Geometry: final body of the model. Coordinates: model frame, mm. A direction names the side the tool comes from. Give positions to 0.01 mm unless a question says otherwise; leave off trailing zeros. Loops run counter-clockwise (first coordinate to the right, second up) from the corner with the lowest first, then second, coordinate; pieces in that order, holes last. Notation, with made-up numbers: (56, -37.75) - (74, -37.75) arc R26 cw to (74, -16.75) - close; hole circle Ø11 at (18, -26.75). An arc over 180 degrees is marked (long way). Answer in a Markdown table with one row per item.
from build123d import *

# Parameters (mm, degrees)
BOSS_EXTRUDE2_DEPTH    = 4
SKETCH4_W              = 35
SKETCH4_H              = 4
BOSS_EXTRUDE3_DEPTH    = 10
BOSS_EXTRUDE4_DEPTH    = 35
SKETCH9_R              = 2.5
CUT_EXTRUDE1_DEPTH     = 6
SKETCH10_R             = 1.25
CUT_EXTRUDE2_DEPTH     = 6
SKETCH11_R             = 2.5
CUT_EXTRUDE3_DEPTH     = 4
CONVERT_SOLID2_START   = -17.5
CONVERT_SOLID2_DEPTH   = 35
CONVERT_SOLID2_2_DEPTH = 35
CONVERT_SOLID2_3_DEPTH = 15
CONVERT_SOLID2_START_2 = 2.5
CONVERT_SOLID2_4_DEPTH = 15


# Read off the part's stored shape, not the designer's step: Convert-Solid2
with BuildPart() as part:
    # Sketch3 → Boss-Extrude2 (new body)
    with BuildSketch(Plane(origin=(0, 0, 0), x_dir=(1, 0, 0), z_dir=(0, 1, 0))):
        with BuildLine():
            Line((-17.5, 0), (-17.5, 27.5))
            Line((-17.5, 27.5), (17.5, 27.5))
            Line((17.5, 27.5), (17.5, 0))
            ThreePointArc((17.5, 0), (0, -17.5), (-17.5, 0))
        make_face()
    extrude(amount=BOSS_EXTRUDE2_DEPTH)

    # Sketch4 → Boss-Extrude3 (add)
    with BuildSketch(Plane(origin=(0, 4, 0), x_dir=(1, 0, 0), z_dir=(0, 1, 0))):
        with Locations((0, 25.5)):
            Rectangle(SKETCH4_W, SKETCH4_H)
    extrude(amount=BOSS_EXTRUDE3_DEPTH)

    # Sketch6 → Boss-Extrude4 (add)
    with BuildSketch(Plane.ZY.offset(17.5)):
        Polygon((-27.5, 14), (-27.5, 18), (-2.5, 18), (-2.5, 128), (1.5, 128), (1.5, 14), align=None)
    extrude(amount=-BOSS_EXTRUDE4_DEPTH)

    # Sketch9 → Cut-Extrude1 (cut)
    with BuildSketch(Plane.XY.offset(1.5)):
        with Locations((-8.9, 117.2)):
            Circle(SKETCH9_R)
        with Locations(Location((8.9, 117.2, 0), (0, 0, 180))):
            Circle(SKETCH9_R)
        with Locations(Location((-8.9, 42.7, 0), (0, 0, 180))):
            Circle(SKETCH9_R)
        with Locations((8.9, 42.7)):
            Circle(SKETCH9_R)
        Polygon((-15.1, 113), (-2.5, 113), (-2.5, 125.287895972), (0, 125.287895972), (2.5, 125.287895972), (2.5, 113), (15.1, 113), (15.1, 46.9), (2.5, 46.9), (2.5, 10), (-2.5, 10), (-2.5, 46.9), (-15.1, 46.9), align=None)
    extrude(amount=-CUT_EXTRUDE1_DEPTH, mode=Mode.SUBTRACT)

    # Sketch10 → Cut-Extrude2 (cut)
    with BuildSketch(Plane.XZ):
        with Locations(Location((-8.75, 0, 0), (0, 0, 270))):
            Circle(SKETCH10_R)
        with Locations(Location((8.75, 0, 0), (0, 0, 90))):
            Circle(SKETCH10_R)
        with Locations(Location((0, 8.75, 0), (0, 0, 270))):
            Circle(SKETCH10_R)
        with Locations(Location((0, -8.75, 0), (0, 0, 270))):
            Circle(SKETCH10_R)
    extrude(amount=-CUT_EXTRUDE2_DEPTH, mode=Mode.SUBTRACT)

    # Sketch11 → Cut-Extrude3 (cut)
    with BuildSketch(Plane.XZ):
        with Locations(Location((0, 0, 0), (0, 0, 270))):
            Circle(SKETCH11_R)
    extrude(amount=-CUT_EXTRUDE3_DEPTH, mode=Mode.SUBTRACT)

    # Convert-Solid2 outline → Convert-Solid2 (cut)
    with BuildSketch(Plane.YZ.offset(CONVERT_SOLID2_START)):
        with BuildLine():
            Line((0, -27.5), (4.1, -27.5))
            ThreePointArc((4.1, -27.5), (1.200862197, -26.299137803), (0, -23.4))
            Line((0, -23.4), (0, -27.5))
        make_face()
        with BuildLine():
            Line((18, -27.5), (18, -23.4))
            ThreePointArc((18, -23.4), (16.799137803, -26.299137803), (13.9, -27.5))
            Line((13.9, -27.5), (18, -27.5))
        make_face()
        with BuildLine():
            ThreePointArc((14, -2.6), (15.200862197, 0.299137803), (18.1, 1.5))
            Line((18.1, 1.5), (14, 1.5))
            Line((14, 1.5), (14, -2.6))
        make_face()
    extrude(amount=CONVERT_SOLID2_DEPTH, mode=Mode.SUBTRACT)

    # Convert-Solid2 2 outline → Convert-Solid2 2 (add)
    with BuildSketch(Plane.YZ.offset(CONVERT_SOLID2_START)):
        with BuildLine():
            Line((4, -23.5), (4.1, -23.5))
            ThreePointArc((4.1, -23.5), (4.029289322, -23.470710678), (4, -23.4))
            Line((4, -23.4), (4, -23.5))
        make_face()
        with BuildLine():
            Line((14, -23.5), (14, -23.4))
            ThreePointArc((14, -23.4), (13.970710678, -23.470710678), (13.9, -23.5))
            Line((13.9, -23.5), (14, -23.5))
        make_face()
    extrude(amount=CONVERT_SOLID2_2_DEPTH)

    # Convert-Solid2 3 outline → Convert-Solid2 3 (add)
    with BuildSketch(Plane.YZ.offset(CONVERT_SOLID2_START)):
        with BuildLine():
            ThreePointArc((18, -2.6), (18.029289322, -2.529289322), (18.1, -2.5))
            Line((18.1, -2.5), (18, -2.5))
            Line((18, -2.5), (18, -2.6))
        make_face()
    extrude(amount=CONVERT_SOLID2_3_DEPTH)

    # Convert-Solid2 4 outline → Convert-Solid2 4 (add)
    with BuildSketch(Plane.YZ.offset(CONVERT_SOLID2_START_2)):
        with BuildLine():
            ThreePointArc((18, -2.6), (18.029289322, -2.529289322), (18.1, -2.5))
            Line((18.1, -2.5), (18, -2.5))
            Line((18, -2.5), (18, -2.6))
        make_face()
    extrude(amount=CONVERT_SOLID2_4_DEPTH)


solid = part.part
Q1. Draft query along X for faces 1 (the flat face through (15.1, 80, 0)), 2 (the flat face through (-17.5, 49, -2)), 3 (the flat face through (0, 14, -13)). Return one class per face: pulls with the +X half, pulls with the -X half, needs draft (parallel to the pull), parting line crosses it, or undercut.
Check values:
| item | result |
|---|---|
| face 1 | undercut |
| face 2 | pulls with the -X half |
| face 3 | needs draft |
Q2. Cut plane A-A (y = 42.7). Output: boundary loops of the cut face in (x, z).
Check values:
| item | result |
|---|---|
| outline | (-17.5, -2.5) - (-11.4, -2.5) - (-11.4, 1.5) - (-17.5, 1.5) - close; (-6.4, -2.5) - (-2.5, -2.5) - (-2.5, 1.5) - (-6.4, 1.5) - close; (2.5, -2.5) - (6.4, -2.5) - (6.4, 1.5) - (2.5, 1.5) - close; (11.4, -2.5) - (17.5, -2.5) - (17.5, 1.5) - (11.4, 1.5) - close |
Q3. Cut plane C-C (y = 67). Output: boundary loops of the cut face in (x, z), and give its area (3 significant figures).
Check values:
| item | result |
|---|---|
| outline | (-17.5, -2.5) - (-15.1, -2.5) - (-15.1, 1.5) - (-17.5, 1.5) - close; (15.1, -2.5) - (17.5, -2.5) - (17.5, 1.5) - (15.1, 1.5) - close |
| area | 19.2 mm² |
Q4. Cut plane D-D (x = 4). Output: boundary loops of the cut face in (y, z).
Check values:
| item | result |
|---|---|
| outline | (0, -23.4) arc R4.1 ccw to (4.1, -27.5) - (13.9, -27.5) arc R4.1 ccw to (18, -23.4) - (18, -2.6) arc R0.1 cw to (18.1, -2.5) - (46.9, -2.5) - (46.9, 1.5) - (18.1, 1.5) arc R4.1 ccw to (14, -2.6) - (14, -23.4) arc R0.1 cw to (13.9, -23.5) - (4.1, -23.5) arc R0.1 cw to (4, -23.4) - (4, 17.04) - (0, 17.04) - close; (113, -2.5) - (128, -2.5) - (128, 1.5) - (113, 1.5) - close |
Q5. Cut plane B-B (z = -13.5). Output: boundary loops of the cut face in (x, y), and give its area (3 significant figures).
Check values:
| item | result |
|---|---|
| outline | (-17.5, 0) - (17.5, 0) - (17.5, 4) - (-17.5, 4) - close; (-17.5, 14) - (17.5, 14) - (17.5, 18) - (-17.5, 18) - close |
| area | 280 mm² |
Q6. Material intervals for line 1 along Y through (x, z) = (11, -3); line 2 along Y through (x, z) = (-8.9, 0.65); line 3 along Y through (x, z) = (-8, 0), sorted ascending.
Check values:
| item | result |
|---|---|
| line 1 | 0 to 4, 14 to 18 |
| line 2 | 15.6 to 40.2, 45.2 to 46.9, 113 to 114.7, 119.7 to 128 |
| line 3 | 14.93 to 40.37, 45.03 to 46.9, 113 to 114.87, 119.53 to 128 |
Q7. Reachability of faces 4 (the flat face through (2.5, 30, -1)), 5 (the flat face through (9, 46.9, 0)), 6 (the cylindrical face through (-10.1, 15.2, 0.3)), 7 (the flat face through (15.3, 61.6, 1.5)) from +Z, -Z, +X, -X, +Y, -Y: full face, straight path, thin tool, end or side. Return the list, or none.
Check values:
| item | result |
|---|---|
| face 4 | +Z |
| face 5 | +Z, -Z |
| face 6 | +Z, +X, -X |
| face 7 | +Z, +X, -X, +Y |
Q8. First-contact query: pin 1 (1.2 mm diameter, centred on x = -1, z = 0.5, fed in from -Y); pin 2 (1.2 mm diameter, centred on x = -1, y = 15, fed in from +Z). Flat tips, straight axial feed; report the tip coordinate or a pass-through.
Check values:
| item | result |
|---|---|
| pin 1 | y = 125.29 |
| pin 2 | z = -4.5 |
